```python
from build123d import *

# Parameters (mm, degrees)
MAIN_BODY_DEPTH         = 5
CONVERT_SOLID1_START    = -5
CONVERT_SOLID1_DEPTH    = 10
CONVERT_SOLID1_2_DEPTH  = 10
SKETCH6_R               = 1.5
MIDDLE_RIVET_HOLE_DEPTH = 14.224598293
SKETCH7_R               = 1.5
LEFT_RIVET_HOLE_DEPTH   = 13.731457104
FILLET1_R               = 3


# Read off the part's stored shape, not the designer's step: Convert-Solid1
with BuildPart() as part:
    # Sketch1 → MAIN BODY (new, symmetric)
    with BuildSketch(Plane.XY):
        Polygon((11.5, 0), (5, 0), (3.25, 2.2), (0, 2.2), (0, 0.2), (2.285328582, 0.2), (4.035328582, -2), (11.5, -2), align=None)
    main_body = extrude(amount=MAIN_BODY_DEPTH, both=True)

    # Mirror1: MAIN BODY across plane
    add(main_body.mirror(Plane(origin=(0, 0, 0), x_dir=(0, 0, 1), z_dir=(1, 0, 0))))

    # Convert-Solid1 outline → Convert-Solid1 (cut)
    with BuildSketch(Plane.XY.offset(CONVERT_SOLID1_START)):
        with BuildLine():
            ThreePointArc((-4.000663363, 1.256308915), (-3.130261025, 1.951751794), (-2.044160728, 2.2))
            Line((-2.044160728, 2.2), (-3.25, 2.2))
            Line((-3.25, 2.2), (-4.000663363, 1.256308915))
        make_face()
        with BuildLine():
            ThreePointArc((2.044160728, 2.2), (3.130261025, 1.951751794), (4.000663363, 1.256308915))
            Line((4.000663363, 1.256308915), (3.25, 2.2))
            Line((3.25, 2.2), (2.044160728, 2.2))
        make_face()
        with BuildLine():
            Line((-4.035328582, -2), (-3.284665219, -1.056308915))
            ThreePointArc((-3.284665219, -1.056308915), (-4.155067557, -1.751751794), (-5.241167854, -2))
            Line((-5.241167854, -2), (-4.035328582, -2))
        make_face()
        with BuildLine():
            ThreePointArc((5.241167854, -2), (4.155067557, -1.751751794), (3.284665219, -1.056308915))
            Line((3.284665219, -1.056308915), (4.035328582, -2))
            Line((4.035328582, -2), (5.241167854, -2))
        make_face()
    extrude(amount=CONVERT_SOLID1_DEPTH, mode=Mode.SUBTRACT)

    # Convert-Solid1 2 outline → Convert-Solid1 2 (add)
    with BuildSketch(Plane.XY.offset(CONVERT_SOLID1_START)):
        with BuildLine():
            Line((-5, 0), (-4.849867327, 0.188738217))
            ThreePointArc((-4.849867327, 0.188738217), (-5.023947795, 0.049649641), (-5.241167854, 0))
            Line((-5.241167854, 0), (-5, 0))
        make_face()
        with BuildLine():
            ThreePointArc((5.241167854, 0), (5.023947795, 0.049649641), (4.849867327, 0.188738217))
            Line((4.849867327, 0.188738217), (5, 0))
            Line((5, 0), (5.241167854, 0))
        make_face()
        with BuildLine():
            ThreePointArc((-2.435461255, 0.011261783), (-2.261380788, 0.150350359), (-2.044160728, 0.2))
            Line((-2.044160728, 0.2), (-2.285328582, 0.2))
            Line((-2.285328582, 0.2), (-2.435461255, 0.011261783))
        make_face()
        with BuildLine():
            ThreePointArc((2.044160728, 0.2), (2.261380788, 0.150350359), (2.435461255, 0.011261783))
            Line((2.435461255, 0.011261783), (2.285328582, 0.2))
            Line((2.285328582, 0.2), (2.044160728, 0.2))
        make_face()
    extrude(amount=CONVERT_SOLID1_2_DEPTH)

    # Sketch6 → MIDDLE RIVET HOLE (cut, through all)
    with BuildSketch(Plane(origin=(0, 2.2, 0), x_dir=(1, 0, 0), z_dir=(0, 1, 0))):
        with Locations(Location((0, 0, 0), (0, 0, 180))):
            Circle(SKETCH6_R)
    extrude(amount=-MIDDLE_RIVET_HOLE_DEPTH, mode=Mode.SUBTRACT)

    # Sketch7 → LEFT RIVET HOLE (cut, through all)
    with BuildSketch(Plane(origin=(0, 0, 0), x_dir=(1, 0, 0), z_dir=(0, 1, 0))):
        with Locations(Location((-9, 0, 0), (0, 0, 180))):
            Circle(SKETCH7_R)
    left_rivet_hole = extrude(amount=-LEFT_RIVET_HOLE_DEPTH, mode=Mode.SUBTRACT)

    # RIGHT RIVET HOLE: LEFT RIVET HOLE across plane
    add(left_rivet_hole.mirror(Plane(origin=(0, 0, 0), x_dir=(0, 0, 1), z_dir=(1, 0, 0))), mode=Mode.SUBTRACT)

    # Fillet1
    fillet1_edges = [part.edges().sort_by_distance(p)[0] for p in [
        (11.5, -1, -5),
        (11.5, -1, 5),
        (-11.5, -1, 5),
        (-11.5, -1, -5),
    ]]
    fillet(fillet1_edges, radius=FILLET1_R)


solid = part.part
```
Geometry check sheet. Reference: the model listing, model coordinates, mm. A direction names the side the tool comes from. Round coordinates to 2 decimals unless told otherwise and drop trailing zeros. Order: outer loops, then holes, each group sorted by start corner. A loop starts at its lowest first (then second) coordinate and runs counter-clockwise, first axis right, second up. Notation, with made-up numbers: (-40, 16.5) - (-26, 16.5) arc R22 ccw to (-26, 50.5) - close; hole circle Ø4 at (17, 18.5). An arc over 180 degrees is marked (long way). Use a Markdown table: item, result. Add a question column.
1) Set-up check for faces 4 (the cylindrical face through (4.17, -1.76, -0.07)), 5 (the cylindrical face through (10.6, -0.99, -4.14)): record each of +Z, -Z, +X, -X, +Y, -Y from which the full face is reachable in a straight line by a thin tool's end or side.
2) Section check A-A (x = 0). Record the cut outline in (y, z), then the cut area to 3 significant figures.
3) Mould release check, pull along Z, two halves, no side actions. Record for faces 1 (the flat face through (0, 1, -5)), 2 (the flat face through (2.854, -0.515, 0.07)), 3 (the cylindrical face through (7.5, -0.99, 0.07)): released by +Z, released by -Z, zero draft, split by the parting line, or undercut.
4) Section check B-B (z = 0). Count the separate pieces of the cut face and the enclosed holes in it, then the cut area to 3 significant figures.
5) Section check C-C (y = -1.35). Record the cut outline in (x, z), then the cut area to 3 significant figures.
6) Thickness scan on line 1 along Z through (x, y) = (0, 1.7); line 2 along Y through (x, z) = (-10.5, -2.25); line 3 along Y through (x, z) = (2, 0.25). Record the ranges inside material, lowest first.
7) Gauge pin test, flat ends, axial feed: P1, Ø2.5, axis at x = 9, z = 0, coming from the -Y side; P2, Ø2, axis at y = 1.5, z = 2.5, coming from the +X side; P3, Ø4, axis at x = 0, z = 0, coming from the -Y side; P4, Ø5, axis at x = -9, z = 0, coming from the +Y side. Record the tip position at first contact, or that the pin passes through.
8) Section check D-D (x = -9). Record the cut outline in (y, z).
Established:
| question | item | result |
|---|---|---|
| 1 | face 4 | +Z, -Z, -Y |
| 1 | face 5 | -Z, +X, +Y, -Y |
| 2 | outline | (0.2, -5) - (2.2, -5) - (2.2, -1.5) - (0.2, -1.5) - close; (0.2, 1.5) - (2.2, 1.5) - (2.2, 5) - (0.2, 5) - close |
| 2 | area | 14.0 mm2 |
| 3 | face 1 | released by -Z |
| 3 | face 2 | zero draft |
| 3 | face 3 | undercut |
| 4 | separate pieces | 4 |
| 4 | enclosed holes | 0 |
| 4 | area | 31.5 mm2 |
| 5 | outline | (-11.5, -2) arc R3 ccw to (-8.5, -5) - (-3.56, -5) - (-3.56, 5) - (-8.5, 5) arc R3 ccw to (-11.5, 2) - close; (3.56, -5) - (8.5, -5) arc R3 ccw to (11.5, -2) - (11.5, 2) arc R3 ccw to (8.5, 5) - (3.56, 5) - close; hole circle Ø3 at (-9, 0); hole circle Ø3 at (9, 0) |
| 5 | area | 137 mm2 |
| 6 | line 1 | -5 to -1.5, 1.5 to 5 |
| 6 | line 2 | -2 to 0 |
| 6 | line 3 | 0.2 to 2.2 |
| 7 | P1 | through |
| 7 | P2 | x = 4.6 |
| 7 | P3 | y = 0.2 |
| 7 | P4 | y = 0 |
| 8 | outline | (-2, -4.96) - (0, -4.96) - (0, -1.5) - (-2, -1.5) - close; (-2, 1.5) - (0, 1.5) - (0, 4.96) - (-2, 4.96) - close |
